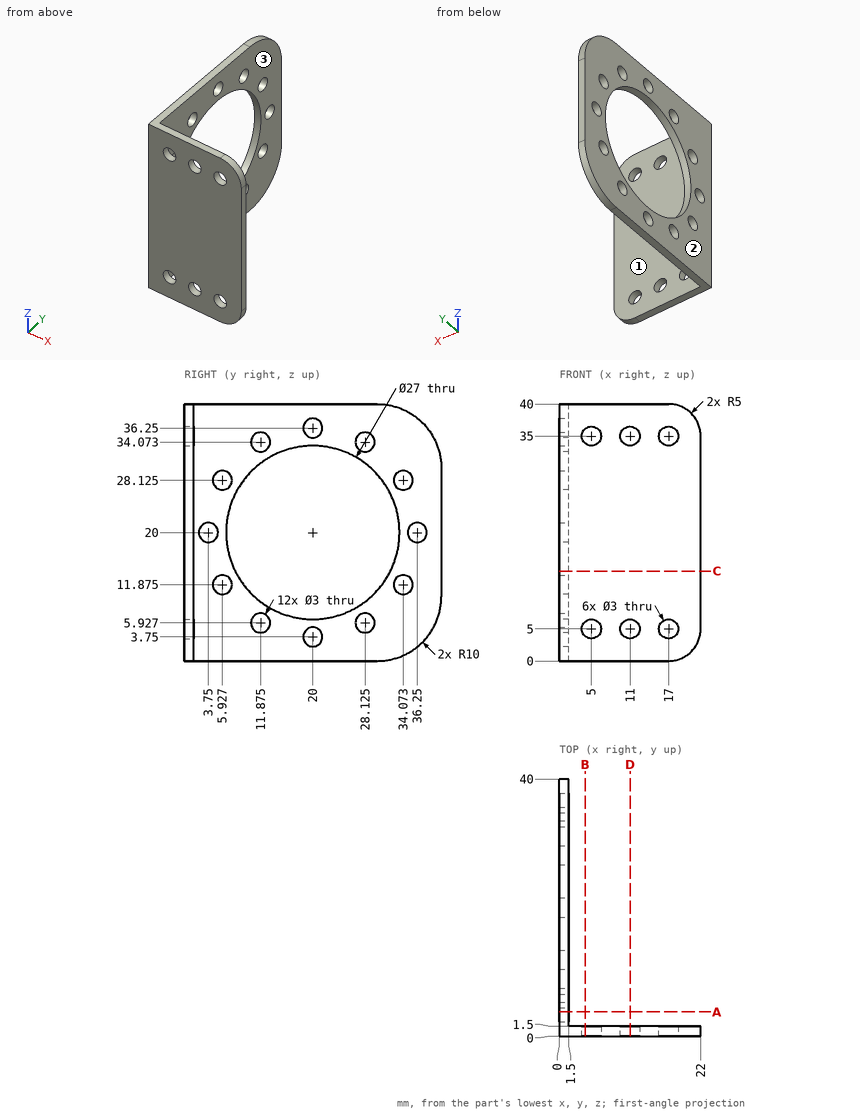
Part print with two shaded views. Sizes in mm from the minimum x, y, z corner. Coordinates: 2 decimals unless noted, no trailing zeros. Order: outer loops, then holes, each group sorted by start corner. A loop starts at its lowest first (then second) coordinate and runs counter-clockwise, first axis right, second up.
(1) Saw through at C-C, the plane z = 14. Write the cut outline in (x, y), and give its area (3 significant figures).
Solution:
outline: (0, 0) - (22, 0) - (22, 1.5) - (1.5, 1.5) - (1.5, 7.91) - (0, 7.91) - close; (0, 32.09) - (1.5, 32.09) - (1.5, 40) - (0, 40) - close
area: 54.5 mm2
(2) Saw through at B-B, the plane x = 4. Write the cut outline in (y, z), and give its area (3 significant figures).
Solution:
outline: (0, 0) - (1.5, 0) - (1.5, 3.88) - (0, 3.88) - close; (0, 6.12) - (1.5, 6.12) - (1.5, 33.88) - (0, 33.88) - close; (0, 36.12) - (1.5, 36.12) - (1.5, 40) - (0, 40) - close
area: 53.3 mm2
(3) Drill centre lines: L1, parallel to Z at x = 5, y = 0.5; L2, parallel to X at y = 1.05, z = 5; L3, parallel to Y at x = 0.85, z = 20. Where is each one in solid material? Low to high.
Solution:
L1: z = 0 to 3.5, 6.5 to 33.5, 36.5 to 40
L2: x = 0 to 3.5, 6.5 to 9.5, 12.5 to 15.5, 18.5 to 22
L3: y = 0 to 2.25, 5.25 to 6.5, 33.5 to 34.75, 37.75 to 40
(4) Saw through at A-A, the plane y = 3.75. Write the cut outline in (x, z), and give its area (3 significant figures).
Solution:
outline: (0, 0) - (1.5, 0) - (1.5, 18.5) - (0, 18.5) - close; (0, 21.5) - (1.5, 21.5) - (1.5, 40) - (0, 40) - close
area: 55.5 mm2
(5) Mould opens along X. For the marked faces 1, 2 and 3 say: released by +X, released by -X, zero draft, split by the parting line, or undercut.
Solution:
face 1: zero draft
face 2: released by -X
face 3: released by +X
(6) Saw through at D-D, the plane x = 11. Write the cut outline in (y, z).
Solution:
outline: (0, 0) - (1.5, 0) - (1.5, 3.5) - (0, 3.5) - close; (0, 6.5) - (1.5, 6.5) - (1.5, 33.5) - (0, 33.5) - close; (0, 36.5) - (1.5, 36.5) - (1.5, 40) - (0, 40) - close
(7) Pin check, flat tips, straight feed: pin 1 Ø2.5 at (y, z) = (5.93, 28.12) entering from +X; pin 2 Ø12 at (y, z) = (9, 13.5) entering from +X; pin 3 Ø1.5 at (x, z) = (10.5, 6.5) entering from +Y. Stop position of each tip, or through.
Solution:
pin 1: passes through
pin 2: stops at x = 1.5
pin 3: stops at y = 1.5
